Design review of the part built by this model. Coordinates are the model's own, in mm. Face numbers are marked on the shaded views. A direction names the side the tool comes from. Coordinates: 2 decimals unless noted, no trailing zeros. Write each loop counter-clockwise with the first axis right and the second up, starting at its lowest first coordinate (ties: lowest second). Pieces come first, ordered by that corner, then holes.
Q1. Take a section at D-D (x = 9). Give the boundary of the cut face in (y, z).
Q2. Insertion check: pin 1 (3 mm diameter, centred on x = -8.5, z = -27, fed in from -Y); pin 2 (9 mm diameter, centred on x = -21, z = -32.5, fed in from -Y); pin 3 (4.5 mm diameter, centred on y = 13.5, z = -31.5, fed in from +X); pin 4 (3 mm diameter, centred on x = -15, y = 10.5, fed in from +Z). Each pin has a flat end and moves straight along its axis. Give the tip position at first contact, or say it passes through.
Q3. Take a section at B-B (x = -21). Give the boundary of the cut face in (y, z), and give its area (3 significant figures).
Q4. Take a section at C-C (y = 6). Give the boundary of the cut face in (x, z), and give its area (3 significant figures).
Q5. Machinability: for the marked faces 1 and 2, which of the approach directions +Z, -Z, +X, -X, +Y, -Y give a long, thin tool a straight path to every point of the face, cutting with its end or side? Answer none if there is none.
Q6. Take a section at A-A (z = -17). Give the boundary of the cut face in (x, y).
Q7. For probe 1 along X at (y, z) = (12.35, -34.5); probe 2 along Z at (x, y) = (0.5, 2.75); probe 3 along X at (y, z) = (13.25, 11.5), list the stretches that pass through material, from the lowest coordinate up.
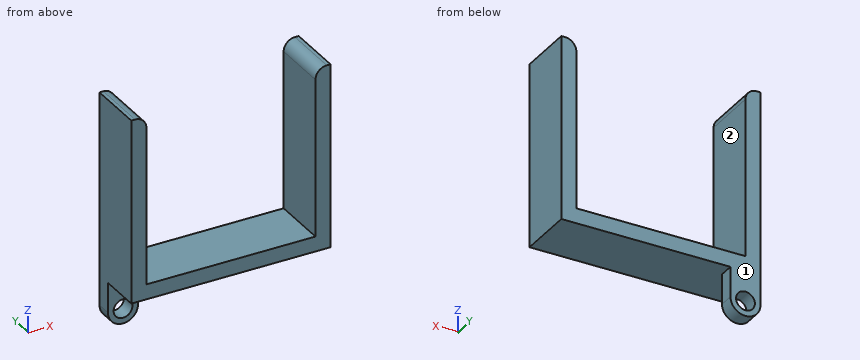
```python
from build123d import *

# Parameters (mm, degrees)
BOSS_EXTRUDE1_DEPTH = 15
FILLET1_R           = 3
SKETCH2_R           = 4
SKETCH2_R_2         = 2.5
BOSS_EXTRUDE2_DEPTH = 4


with BuildPart() as part:
    # Sketch1 → Boss-Extrude1 (new body)
    with BuildSketch(Plane(origin=(0, 0, 0), x_dir=(1, 0, 0), z_dir=(0, 1, 0))):
        Polygon((22.5, -22.5), (22.5, 22.5), (-22.5, 22.5), (-22.5, -22.5), (-26.5, -22.5), (-26.5, 26.5), (26.5, 26.5), (26.5, -22.5), align=None)
    extrude(amount=BOSS_EXTRUDE1_DEPTH)

    # Fillet1
    fillet1_edges = [part.edges().sort_by_distance(p)[0] for p in [
        (-22.5, 7.5, 22.5),
        (22.5, 7.5, 22.5),
    ]]
    fillet(fillet1_edges, radius=FILLET1_R)

    # Sketch2 → Boss-Extrude2 (add)
    # profile 1 of 2: a face of its own
    with BuildSketch(Plane(origin=(0, 15, 0), x_dir=(1, 0, 0), z_dir=(0, 1, 0))):
        with Locations((-22.5, 34.5)):
            Circle(SKETCH2_R)
        with Locations(Location((-22.5, 34.5, 0), (0, 0, 270))):
            Circle(SKETCH2_R_2, mode=Mode.SUBTRACT)
    # profile 2 of 2: a face of its own
    with BuildSketch(Plane(origin=(0, 15, 0), x_dir=(1, 0, 0), z_dir=(0, 1, 0))):
        with BuildLine():
            Line((-18.5, 26.5), (-18.5, 34.5))
            ThreePointArc((-18.5, 34.5), (-22.5, 30.5), (-26.5, 34.5))
            Line((-26.5, 34.5), (-26.5, 26.5))
            Line((-26.5, 26.5), (-18.5, 26.5))
        make_face()
    extrude(amount=-BOSS_EXTRUDE2_DEPTH)


solid = part.part
```
Response:
1. outline: (0, -26.5) - (15, -26.5) - (15, -22.5) - (0, -22.5) - close
2. pin 1: stops at y = 0
2. pin 2: stops at y = 11
2. pin 3: stops at x = -18.5
2. pin 4: stops at z = -22.5
3. outline: (0, -26.5) - (11, -26.5) - (11, -32.5) - (15, -32.5) - (15, -22.5) - (0, -22.5) - close; (11, -38.21) - (15, -38.21) - (15, -36.5) - (11, -36.5) - close
3. area: 90.8 mm2
4. outline: (-26.5, -26.5) - (26.5, -26.5) - (26.5, 22.5) - (25.5, 22.5) arc R3 ccw to (22.5, 19.5) - (22.5, -22.5) - (-22.5, -22.5) - (-22.5, 19.5) arc R3 ccw to (-25.5, 22.5) - (-26.5, 22.5) - close
4. area: 568 mm2
5. face 1: +Z, -Z, +X, -X, +Y
5. face 2: +Z, +Y, -Y
6. outline: (-26.5, 0) - (-22.5, 0) - (-22.5, 15) - (-26.5, 15) - close; (22.5, 0) - (26.5, 0) - (26.5, 15) - (22.5, 15) - close
7. probe 1: x = -26.5 to -25, -20 to -18.5
7. probe 2: z = -26.5 to -22.5
7. probe 3: x = -26.5 to -22.5, 22.5 to 26.5
